from build123d import *

# Parameters (mm, degrees)
SKETCH1_R           = 50
SKETCH1_R_2         = 3
SKETCH1_R_3         = 1.5
SKETCH1_R_4         = 1.75
BOSS_EXTRUDE1_DEPTH = 3
SKETCH2_R           = 5
CUT_EXTRUDE1_DEPTH  = 2
CHAMFER1_SIZE       = 1


with BuildPart() as part:
    # Sketch1 → Boss-Extrude1 (new body)
    with BuildSketch(Plane(origin=(0, 0, 0), x_dir=(1, 0, 0), z_dir=(0, 1, 0))):
        with Locations(Location((0, 0, 0), (0, 0, 270))):
            Circle(SKETCH1_R)
        with Locations(Location((0, 0, 0), (0, 0, 270))):
            Circle(SKETCH1_R_2, mode=Mode.SUBTRACT)
        with Locations(Location((-39.8, -22.978540714, 0), (0, 0, 270))):
            Circle(SKETCH1_R_3, mode=Mode.SUBTRACT)
        with Locations(Location((-17.45, -7.989233767, 0), (0, 0, 270))):
            Circle(SKETCH1_R_4, mode=Mode.SUBTRACT)
        with Locations(Location((0, 45.95, 0), (0, 0, 270))):
            Circle(SKETCH1_R_3, mode=Mode.SUBTRACT)
        with Locations(Location((0, -38.0178, 0), (0, 0, 270))):
            Circle(SKETCH1_R_4, mode=Mode.SUBTRACT)
        with Locations(Location((39.8, -22.978540714, 0), (0, 0, 90))):
            Circle(SKETCH1_R_3, mode=Mode.SUBTRACT)
        with Locations(Location((17.45, -7.989233767, 0), (0, 0, 90))):
            Circle(SKETCH1_R_4, mode=Mode.SUBTRACT)
    extrude(amount=BOSS_EXTRUDE1_DEPTH)

    # Sketch2 → Cut-Extrude1 (cut)
    with BuildSketch(Plane(origin=(0, 3, 0), x_dir=(1, 0, 0), z_dir=(0, 1, 0))):
        with Locations(Location((0, 0, 0), (0, 0, 270))):
            Circle(SKETCH2_R)
    extrude(amount=-CUT_EXTRUDE1_DEPTH, mode=Mode.SUBTRACT)

    # Chamfer1
    chamfer1_edges = [part.edges().sort_by_distance(p)[0] for p in [
        (0, 0, -47.45),
        (39.8, 0, 24.478540714),
        (-39.8, 0, 21.478540714),
    ]]
    chamfer(chamfer1_edges, length=CHAMFER1_SIZE)


solid = part.part
Design review of the part built by this model. Coordinates are the model's own, in mm. A direction names the side the tool comes from. Round coordinates to 2 decimals unless told otherwise and drop trailing zeros. Write each loop counter-clockwise with the first axis right and the second up, starting at its lowest first coordinate (ties: lowest second). Pieces come first, ordered by that corner, then holes. Notation, with made-up numbers: (-28.75, 34) - (25.25, 34) arc R22 ccw to (25.25, 42) - close; hole circle Ø8 at (27, 8.5). An arc over 180 degrees is marked (long way). Use a Markdown table: item, result. Add a question column.
1. We need section D-D (z = -14). State the section outline as (x, y) points, then the cut area to 3 significant figures.
2. Mouldability with a two-part tool opening along X and no side actions: class faces 1 (the face through (1, 0, 10)), 2 (the face through (15.02, 1.48, 47.69)), 3 (the face through (16.27, 1.48, 9.28)) as +X half, -X half, draft (parallel to the pull), parting line (faces both ways), or undercut.
3. Clearance check with flat-ended pins moving along their axes: pin 1 (4.5 mm diameter, centred on x = 17.45, z = 7.99, fed in from -Y); pin 2 (5 mm diameter, centred on x = 0, z = 1.5, fed in from +Y); pin 3 (1.8 mm diameter, centred on x = 0, z = -45.95, fed in from -Y); pin 4 (1 mm diameter, centred on y = 1, z = -36.5, fed in from -X). State where each tip first meets the part, or that it passes through.
4. Wall thickness on probe 1 along Z at (x, y) = (39.8, 1.9); probe 2 along X at (y, z) = (2.05, 1); probe 3 along X at (y, z) = (1.6, 28.5): over which ranges is each line inside the solid? List them lowest first.
5. For faces 4 (the face through (-3.3, 1, -0.1)), 5 (the face through (-38.313, 1.986, 22.783)), list the 3-axis set-ups (+Z, -Z, +X, -X, +Y, -Y) from which the entire face can be reached by the end or side of a thin tool; tool diameter is ignored.
6. We need section A-A (y = 2.4). State the section outline as (x, z) points, then the cut area to 3 significant figures.
7. We need section C-C (x = 17.45). State the section outline as (y, z) points, then the cut area to 3 significant figures.
8. We need section B-B (z = 1). State the section outline as (x, y) points.
Output:
| question | item | result |
|---|---|---|
| 1 | outline | (-48, 0) - (48, 0) - (48, 3) - (-48, 3) - close |
| 1 | area | 288 mm2 |
| 2 | face 1 | draft |
| 2 | face 2 | parting line |
| 2 | face 3 | undercut |
| 3 | pin 1 | stops at y = 0 |
| 3 | pin 2 | stops at y = 1 |
| 3 | pin 3 | passes through |
| 3 | pin 4 | stops at x = -34.7 |
| 4 | probe 1 | z = -30.26 to 21.48, 24.48 to 30.26 |
| 4 | probe 2 | x = -49.99 to -4.9, 4.9 to 49.99 |
| 4 | probe 3 | x = -41.08 to 41.08 |
| 5 | face 4 | +Y |
| 5 | face 5 | +Y, -Y |
| 6 | outline | circle Ø100 at (0, 0); hole circle Ø3 at (-39.8, 22.98); hole circle Ø3.5 at (-17.45, 7.99); hole circle Ø10 at (0, 0); hole circle Ø3.5 at (0, 38.02); hole circle Ø3 at (0, -45.95); hole circle Ø3.5 at (17.45, 7.99); hole circle Ø3 at (39.8, 22.98) |
| 6 | area | 7,730 mm2 |
| 7 | outline | (0, -46.86) - (3, -46.86) - (3, 6.24) - (0, 6.24) - close; (0, 9.74) - (3, 9.74) - (3, 46.86) - (0, 46.86) - close |
| 7 | area | 271 mm2 |
| 8 | outline | (-49.99, 0) - (-2.83, 0) - (-2.83, 1) - (-4.9, 1) - (-4.9, 3) - (-49.99, 3) - close; (2.83, 0) - (49.99, 0) - (49.99, 3) - (4.9, 3) - (4.9, 1) - (2.83, 1) - close |
